Geometry: final body of the model. Coordinates: model frame, mm. Round coordinates to 2 decimals unless told otherwise and drop trailing zeros. Write each loop counter-clockwise with the first axis right and the second up, starting at its lowest first coordinate (ties: lowest second). Pieces come first, ordered by that corner, then holes. Notation, with made-up numbers: (84.25, 60) -> (94.25, 60) arc R18 ccw to (94.25, 83) -> close; hole circle Ø10 at (64, 68.25). An arc over 180 degrees is marked (long way). Use one line per item in the form item = value. Start each with the question number.
1. Line query: L1, parallel to Z at x = 23, y = 20.5; L2, parallel to X at y = 7, z = 30; L3, parallel to X at y = 10.5, z = 51.5. Output: solid intervals per line, ascending.
2. Cut plane B-B, the plane z = 37.5. Return the cut outline in (x, y) (3 decimals).
3. Cut plane A-A, the plane y = 25. State how many separate pieces and enclosed holes the cut face has, plus the area to 3 significant figures.
4. Pin query (flat end, axial travel): pin 1 Ø12 at (x, y) = (185.5, 16) entering from +Z; pin 2 Ø8 at (y, z) = (12, 35) entering from +X; pin 3 Ø6 at (x, y) = (220, 37) entering from +Z. Return the tip coordinate at first contact, or that it passes through.
5. Cut plane C-C, the plane x = 153. Return the cut outline in (y, z) (3 decimals).
```python
from build123d import *

# Parameters (mm, degrees)
F1_DEPTH  = 41.275
F2_R      = 9.525
F3_DEPTH  = 50.8
F5_DEPTH  = 50.8
F7_DEPTH  = 50.8
F9_DEPTH  = 50.8
F10_R     = 3.175
F10_R_2   = 3.361139
F11_DEPTH = 228.6
F12_DEPTH = 228.6


with BuildPart() as f1:
    # F0 (on Front) → F1 (new body)
    with BuildSketch(Plane.XZ):
        Polygon((304.8, 19.05), (0, 73.025), (0, 0), (304.8, 0), align=None)
    extrude(amount=-F1_DEPTH)

    # F2 (on face) → F3 (cut)
    with BuildSketch(Plane(origin=(0, 0, 0), x_dir=(0, -1, 0), z_dir=(-1, 0, 0))):
        with Locations((-20.6375, 30.160377)):
            Circle(F2_R)
    extrude(amount=-F3_DEPTH, mode=Mode.SUBTRACT)

    # F4 (on face) → F5 (cut)
    with BuildSketch(Plane.XZ):
        Polygon((0, 73.025), (0, 54.048669), (107.16046, 54.048669), align=None)
        Polygon((253.724616, 28.094599), (107.16046, 54.048669), (120.438509, 27.69807), align=None)
        Polygon((304.8, 19.05), (253.724616, 28.094599), (304.8, 0), align=None)
    extrude(amount=-F5_DEPTH, mode=Mode.SUBTRACT)

    # F6 (on face) → F7 (cut)
    with BuildSketch(Plane.XZ):
        Polygon((63.578897, 27.528911), (120.438509, 27.69807), (107.16046, 54.048669), (63.5, 54.048669), align=None)
    extrude(amount=-F7_DEPTH, mode=Mode.SUBTRACT)

    # F8 (on face) → F9 (cut)
    with BuildSketch(Plane.XZ):
        Polygon((254, 0), (304.8, 0), (253.724616, 28.094599), (206.078957, 27.952852), align=None)
    extrude(amount=-F9_DEPTH, mode=Mode.SUBTRACT)

    # F10 (on face) → F11 (cut)
    with BuildSketch(Plane.XZ):
        with Locations((37.127063, 9.212729)):
            Circle(F10_R)
        with Locations((289.942942, 6.520301)):
            Circle(F10_R_2)
    extrude(amount=-F11_DEPTH, mode=Mode.SUBTRACT)

    # F10 (on face) → F12 (cut)
    with BuildSketch(Plane.XZ):
        with Locations((37.127063, 9.212729)):
            Circle(F10_R)
        with Locations((289.942942, 6.520301)):
            Circle(F10_R_2)
        with Locations((199.063465, 7.915162)):
            Circle(F10_R)
    extrude(amount=-F12_DEPTH, mode=Mode.SUBTRACT)


solid = f1.part
```
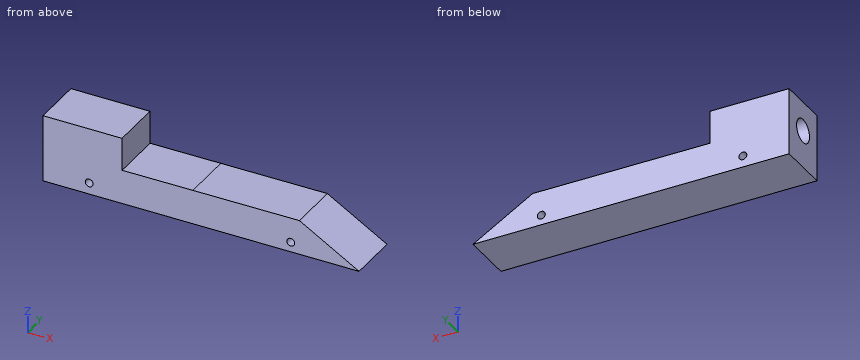
Outcome:
q1.L1 = 0 to 20.64, 39.68 to 54.05
q1.L2 = 0 to 63.57
q1.L3 = 0 to 63.51
q2.outline = (0, 0) -> (63.549, 0) -> (63.549, 41.275) -> (0, 41.275) -> (0, 26.708) -> (50.8, 26.708) -> (50.8, 14.567) -> (0, 14.567) -> close
q3.separate_pieces = 1
q3.enclosed_holes = 2
q3.area = 7,130 mm^2
q4.pin_1 = 27.91
q4.pin_2 = 63.57
q4.pin_3 = 21.58
q5.outline = (0, 0) -> (41.275, 0) -> (41.275, 27.795) -> (0, 27.795) -> close
